Can you work these out from the model? Positions are in its coordinate system, mm. Give positions to 0.01 mm unless a question says otherwise; leave off trailing zeros. Loops run counter-clockwise (first coordinate to the right, second up) from the corner with the lowest first, then second, coordinate; pieces in that order, holes last. Notation, with made-up numbers: (-30, -28.5) - (21, -28.5) arc R17 cw to (21, -17.5) - close; hole circle Ø6 at (49.25, 65.5). An arc over 180 degrees is marked (long way). Answer as a JSON object with one key per item and string values.
```python
from build123d import *

# Parameters (mm, degrees)
SCHIZZO1_W                             = 500
SCHIZZO1_H                             = 600
ESTRUSIONE_ESTRUSIONE1_DEPTH           = 4
SCHIZZO2_W                             = 30
SCHIZZO2_H                             = 100
TAGLIO_ESTRUSIONE1_DEPTH               = 391.532969159
SCHIZZO3_W                             = 29.486887837
SCHIZZO3_H                             = 100
TAGLIO_ESTRUSIONE2_DEPTH               = 391.532969159
TAGLIO_ESTRUSIONE3_DEPTH               = 391.532969159
TAGLIO_ESTRUSIONE4_DEPTH               = 391.532969159
TAGLIO_ESTRUSIONE5_DEPTH               = 391.532969159
TAGLIO_ESTRUSIONE6_DEPTH               = 391.532969159
TAGLIO_ESTRUSIONE7_DEPTH               = 391.532969159
SFORMO1_ANGLE                          = 40.292427289
SFORMO2_ANGLE                          = 39.805571092
FORO_4_5_4_5_1_D                       = 4.5
FORO_SVASATO_PER_VITE_M4_1_AT_2_COUNT  = 2
FORO_SVASATO_PER_VITE_M4_1_AT_2_PITCH  = 150
FORO_SVASATO_PER_VITE_M4_1_AT_3_COUNT  = 2
FORO_SVASATO_PER_VITE_M4_1_AT_3_PITCH  = 300
FORO_SVASATO_PER_VITE_M4_1_AT_4_COUNT  = 2
FORO_SVASATO_PER_VITE_M4_1_AT_4_PITCH  = 450
FORO_SVASATO_PER_VITE_M4_1_AT_5_COUNT  = 2
FORO_SVASATO_PER_VITE_M4_1_AT_5_PITCH  = 370
FORO_SVASATO_PER_VITE_M4_1_AT_6_COUNT  = 2
FORO_SVASATO_PER_VITE_M4_1_AT_6_PITCH  = 399.249295554
FORO_SVASATO_PER_VITE_M4_1_AT_7_COUNT  = 2
FORO_SVASATO_PER_VITE_M4_1_AT_7_PITCH  = 476.340214553
FORO_SVASATO_PER_VITE_M4_1_AT_8_COUNT  = 2
FORO_SVASATO_PER_VITE_M4_1_AT_8_PITCH  = 582.580466545
FORO_SVASATO_PER_VITE_M4_1_AT_9_COUNT  = 2
FORO_SVASATO_PER_VITE_M4_1_AT_9_PITCH  = 105.948100502
FORO_SVASATO_PER_VITE_M4_1_AT_10_COUNT = 2
FORO_SVASATO_PER_VITE_M4_1_AT_10_PITCH = 272.259067801
FORO_SVASATO_PER_VITE_M4_1_AT_11_COUNT = 2
FORO_SVASATO_PER_VITE_M4_1_AT_11_PITCH = 289.698118737
FORO_SVASATO_PER_VITE_M4_1_AT_12_COUNT = 2
FORO_SVASATO_PER_VITE_M4_1_AT_12_PITCH = 145
SMUSSO1_SIZE                           = 5
RACCORDO1_R                            = 1.5
RACCORDO2_R                            = 10


with BuildPart() as part:
    # Schizzo1 → Estrusione-Estrusione1 (new body)
    with BuildSketch(Plane.XY.offset(4)):
        Rectangle(SCHIZZO1_W, SCHIZZO1_H)
    extrude(amount=-ESTRUSIONE_ESTRUSIONE1_DEPTH)

    # Schizzo2 → Taglio-Estrusione1 (cut, through all)
    with BuildSketch(Plane(origin=(0, 0, 0), x_dir=(-1, 0, 0), z_dir=(0, 0, -1))):
        with Locations((235, 0)):
            Rectangle(SCHIZZO2_W, SCHIZZO2_H)
    extrude(amount=-TAGLIO_ESTRUSIONE1_DEPTH, mode=Mode.SUBTRACT)

    # Schizzo3 → Taglio-Estrusione2 (cut, through all)
    with BuildSketch(Plane(origin=(0, 0, 0), x_dir=(-1, 0, 0), z_dir=(0, 0, -1))):
        with Locations((-235.256556082, 0)):
            Rectangle(SCHIZZO3_W, SCHIZZO3_H)
    extrude(amount=-TAGLIO_ESTRUSIONE2_DEPTH, mode=Mode.SUBTRACT)

    # Schizzo4 → Taglio-Estrusione3 (cut, through all)
    with BuildSketch(Plane.XY.offset(4)):
        Polygon((-145, -180), (145, -180), (145, -130), (80, -130), (80, -80), (-81, -80), (-81, -130), (-145, -130), align=None)
    extrude(amount=-TAGLIO_ESTRUSIONE3_DEPTH, mode=Mode.SUBTRACT)

    # Schizzo5 → Taglio-Estrusione4 (cut, through all)
    with BuildSketch(Plane.XY.offset(4)):
        with BuildLine():
            Line((10, -10), (10, 70))
            ThreePointArc((10, 70), (0, 80), (-10, 70))
            Line((-10, 70), (-10, -10))
            ThreePointArc((-10, -10), (0, -20), (10, -10))
        make_face()
    extrude(amount=-TAGLIO_ESTRUSIONE4_DEPTH, mode=Mode.SUBTRACT)

    # Schizzo6 → Taglio-Estrusione5 (cut, through all)
    with BuildSketch(Plane.XY.offset(4)):
        with BuildLine():
            Line((-101, 162.25), (-106, 162.25))
            ThreePointArc((-106, 162.25), (-108.25, 160), (-106, 157.75))
            Line((-106, 157.75), (-101, 157.75))
            ThreePointArc((-101, 157.75), (-98.75, 160), (-101, 162.25))
        make_face()
    extrude(amount=-TAGLIO_ESTRUSIONE5_DEPTH, mode=Mode.SUBTRACT)

    # Schizzo7 → Taglio-Estrusione6 (cut, through all)
    with BuildSketch(Plane.XY.offset(4)):
        with BuildLine():
            Line((-101, 192.25), (-106, 192.25))
            ThreePointArc((-106, 192.25), (-108.25, 190), (-106, 187.75))
            Line((-106, 187.75), (-101, 187.75))
            ThreePointArc((-101, 187.75), (-98.75, 190), (-101, 192.25))
        make_face()
    extrude(amount=-TAGLIO_ESTRUSIONE6_DEPTH, mode=Mode.SUBTRACT)

    # Schizzo8 → Taglio-Estrusione7 (cut, through all)
    with BuildSketch(Plane(origin=(0, 0, 0), x_dir=(-1, 0, 0), z_dir=(0, 0, -1))):
        Polygon((65, 200), (65, 210), (51, 210), (51, 200), (-80, 200), (-80, 150), (51, 150), (51, 140), (65, 140), (65, 150), (96, 150), (96, 200), align=None)
    extrude(amount=-TAGLIO_ESTRUSIONE7_DEPTH, mode=Mode.SUBTRACT)

    # Sformo1
    sformo1_faces = [part.faces().sort_by_distance(p)[0] for p in [
        (235.256556082, 50, 2),
        (235.256556082, -50, 2),
    ]]
    draft(sformo1_faces, Plane(origin=(220.513112163, -50, 4), x_dir=(0, 0, 1), z_dir=(1, 0, 0)), SFORMO1_ANGLE)

    # Sformo2
    sformo2_faces = [part.faces().sort_by_distance(p)[0] for p in [
        (-235, -50, 2),
        (-235, 50, 2),
    ]]
    draft(sformo2_faces, Plane(origin=(-220, 50, 4), x_dir=(0, -1, 0), z_dir=(-1, 0, 0)), SFORMO2_ANGLE)

    # Foro Ø4.5 (4.5)-1 (through all)
    with Locations(Plane.XY.offset(4)):
        with Locations((110, 90), (-110, 90), (110, 30), (-110, 30), (-91, -120), (-91, -90), (89, -120), (89, -90), (90, 190), (90, 160)):
            Hole(FORO_4_5_4_5_1_D / 2)

    # Schizzo11 → Foro svasato per Vite M4-1 (revolve, cut)
    with BuildSketch(Plane(origin=(-185, -175, 4), x_dir=(0, -1, 0), z_dir=(1, 0, 0))):
        Polygon((0, 0), (0, 4), (2.25, 4), (2.25, 2.45), (4.7, 0), align=None)
    foro_svasato_per_vite_m4_1 = revolve(axis=Axis((-185, -175, 10.35), (0, 0, -1)), mode=Mode.SUBTRACT)

    # Foro svasato per Vite M4-1 at 2: Foro svasato per Vite M4-1 ×2
    with Locations(*[(0, i * FORO_SVASATO_PER_VITE_M4_1_AT_2_PITCH, 0) for i in range(1, FORO_SVASATO_PER_VITE_M4_1_AT_2_COUNT)]):
        add(foro_svasato_per_vite_m4_1, mode=Mode.SUBTRACT)

    # Foro svasato per Vite M4-1 at 3: Foro svasato per Vite M4-1 ×2
    with Locations(*[(0, i * FORO_SVASATO_PER_VITE_M4_1_AT_3_PITCH, 0) for i in range(1, FORO_SVASATO_PER_VITE_M4_1_AT_3_COUNT)]):
        add(foro_svasato_per_vite_m4_1, mode=Mode.SUBTRACT)

    # Foro svasato per Vite M4-1 at 4: Foro svasato per Vite M4-1 ×2
    with Locations(*[(0, i * FORO_SVASATO_PER_VITE_M4_1_AT_4_PITCH, 0) for i in range(1, FORO_SVASATO_PER_VITE_M4_1_AT_4_COUNT)]):
        add(foro_svasato_per_vite_m4_1, mode=Mode.SUBTRACT)

    # Foro svasato per Vite M4-1 at 5: Foro svasato per Vite M4-1 ×2
    with Locations(*[(i * FORO_SVASATO_PER_VITE_M4_1_AT_5_PITCH, 0, 0) for i in range(1, FORO_SVASATO_PER_VITE_M4_1_AT_5_COUNT)]):
        add(foro_svasato_per_vite_m4_1, mode=Mode.SUBTRACT)

    # Foro svasato per Vite M4-1 at 6: Foro svasato per Vite M4-1 ×2
    with Locations(*[Vector(0.9267392682234048, 0.37570510873921886, 0) * (i * FORO_SVASATO_PER_VITE_M4_1_AT_6_PITCH) for i in range(1, FORO_SVASATO_PER_VITE_M4_1_AT_6_COUNT)]):
        add(foro_svasato_per_vite_m4_1, mode=Mode.SUBTRACT)

    # Foro svasato per Vite M4-1 at 7: Foro svasato per Vite M4-1 ×2
    with Locations(*[Vector(0.7767557487195029, 0.6298019584212203, 0) * (i * FORO_SVASATO_PER_VITE_M4_1_AT_7_PITCH) for i in range(1, FORO_SVASATO_PER_VITE_M4_1_AT_7_COUNT)]):
        add(foro_svasato_per_vite_m4_1, mode=Mode.SUBTRACT)

    # Foro svasato per Vite M4-1 at 8: Foro svasato per Vite M4-1 ×2
    with Locations(*[Vector(0.6351053995925638, 0.7724254859909594, 0) * (i * FORO_SVASATO_PER_VITE_M4_1_AT_8_PITCH) for i in range(1, FORO_SVASATO_PER_VITE_M4_1_AT_8_COUNT)]):
        add(foro_svasato_per_vite_m4_1, mode=Mode.SUBTRACT)

    # Foro svasato per Vite M4-1 at 9: Foro svasato per Vite M4-1 ×2
    with Locations(*[Vector(0.9438583563660176, -0.33035042472810594, 0) * (i * FORO_SVASATO_PER_VITE_M4_1_AT_9_PITCH) for i in range(1, FORO_SVASATO_PER_VITE_M4_1_AT_9_COUNT)]):
        add(foro_svasato_per_vite_m4_1, mode=Mode.SUBTRACT)

    # Foro svasato per Vite M4-1 at 10: Foro svasato per Vite M4-1 ×2
    with Locations(*[Vector(0.9917025066621883, -0.12855402864139467, 0) * (i * FORO_SVASATO_PER_VITE_M4_1_AT_10_PITCH) for i in range(1, FORO_SVASATO_PER_VITE_M4_1_AT_10_COUNT)]):
        add(foro_svasato_per_vite_m4_1, mode=Mode.SUBTRACT)

    # Foro svasato per Vite M4-1 at 11: Foro svasato per Vite M4-1 ×2
    with Locations(*[Vector(0.9320046715412964, -0.36244626115494755, 0) * (i * FORO_SVASATO_PER_VITE_M4_1_AT_11_PITCH) for i in range(1, FORO_SVASATO_PER_VITE_M4_1_AT_11_COUNT)]):
        add(foro_svasato_per_vite_m4_1, mode=Mode.SUBTRACT)

    # Foro svasato per Vite M4-1 at 12: Foro svasato per Vite M4-1 ×2
    with Locations(*[Vector(0.6896551724137958, -0.7241379310344802, 0) * (i * FORO_SVASATO_PER_VITE_M4_1_AT_12_PITCH) for i in range(1, FORO_SVASATO_PER_VITE_M4_1_AT_12_COUNT)]):
        add(foro_svasato_per_vite_m4_1, mode=Mode.SUBTRACT)

    # Smusso1
    smusso1_edges = [part.edges().sort_by_distance(p)[0] for p in [
        (250, -300, 2),
        (-250, -300, 2),
        (-250, 300, 2),
        (250, 300, 2),
    ]]
    chamfer(smusso1_edges, length=SMUSSO1_SIZE)

    # Raccordo1
    raccordo1_edges = [part.edges().sort_by_distance(p)[0] for p in [
        (-96, 200, 2),
        (-96, 150, 2),
        (-65, 140, 2),
        (-51, 140, 2),
        (80, 150, 2),
        (80, 200, 2),
        (-51, 210, 2),
        (-65, 210, 2),
        (-145, -180, 2),
        (-145, -130, 2),
        (-81, -80, 2),
        (80, -80, 2),
        (145, -130, 2),
        (145, -180, 2),
    ]]
    fillet(raccordo1_edges, radius=RACCORDO1_R)

    # Raccordo2
    raccordo2_edges = [part.edges().sort_by_distance(p)[0] for p in [
        (-250, -75, 2),
        (-220, -50, 2),
        (-220, 50, 2),
        (-250, 75, 2),
        (250, 75, 2),
        (220.513112163, 50, 2),
        (220.513112163, -50, 2),
        (250, -75, 2),
    ]]
    fillet(raccordo2_edges, radius=RACCORDO2_R)


solid = part.part
```
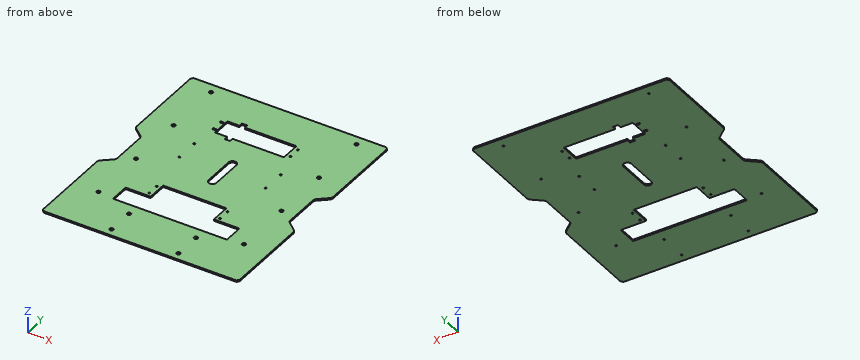
1) Imagine slicing it at A-A on x = 0. Write out the boundary of the cut face in (y, z).
Check sheet entries:
{"outline": "(-300, 0) - (-180, 0) - (-180, 4) - (-300, 4) - close; (-80, 0) - (-20, 0) - (-20, 4) - (-80, 4) - close; (80, 0) - (150, 0) - (150, 4) - (80, 4) - close; (200, 0) - (300, 0) - (300, 4) - (200, 4) - close"}
2) Imagine slicing it at D-D on z = 3.2. Give the number of separate pieces and of enclosed holes in the cut face, and give its area (3 significant figures).
Check sheet entries:
{"separate pieces": "1", "enclosed holes": "27", "area": "258,000 mm2"}
3) I'm going to push flat-ended pins straight in: P1, Ø6, axis at x = -85, y = -280, coming from the +Z side; P2, Ø3.5, axis at x = 85, y = -280, coming from the +Z side; P3, Ø7, axis at x = -110, y = 30, coming from the -Z side. Where does each tip first touch, or does it pass through?
Check sheet entries:
{"P1": "z = 2.3", "P2": "through", "P3": "z = 0"}
4) Imagine slicing it at C-C on x = -123. Write out the boundary of the cut face in (y, z), and give its area (3 significant figures).
Check sheet entries:
{"outline": "(-300, 0) - (-180, 0) - (-180, 4) - (-300, 4) - close; (-130, 0) - (300, 0) - (300, 4) - (-130, 4) - close", "area": "2,200 mm2"}
5) Imagine slicing it at B-B on y = 11. Write out the boundary of the cut face in (x, z).
Check sheet entries:
{"outline": "(-220, 0) - (-10, 0) - (-10, 4) - (-220, 4) - close; (10, 0) - (220.51, 0) - (220.51, 4) - (10, 4) - close"}
6) I need wall thicknesses on L1, parallel to Y at x = -185, z = 1.25; L2, parallel to X at y = -175, z = 0.6; L3, parallel to Y at x = 85, z = 1.05. Which ranges of each line are inside material? Lowest first, please.
Check sheet entries:
{"L1": "-300 to -177.25, -172.75 to -27.25, -22.75 to 122.75, 127.25 to 272.75, 277.25 to 300", "L2": "-250 to -187.25, -182.75 to -145, 145 to 182.75, 187.25 to 250", "L3": "-300 to -282.25, -277.75 to -212.25, -207.75 to -180, -130 to 300"}
